The drawing under review shows one solid part. Ordinate dimensions are in mm from its lowest x, y, z. Give positions to 0.01 mm unless a question says otherwise; leave off trailing zeros. Loops run counter-clockwise (first coordinate to the right, second up) from the corner with the lowest first, then second, coordinate; pieces in that order, holes last. Notation, with made-up numbers: M 35,-31.75 L 91,-31.75 A17 cw 91,-14.75 Z; hole C 14.25,26 d1. An arc over 180 degrees is marked long. Put each result on its own line as item: value. Start each with the question number.
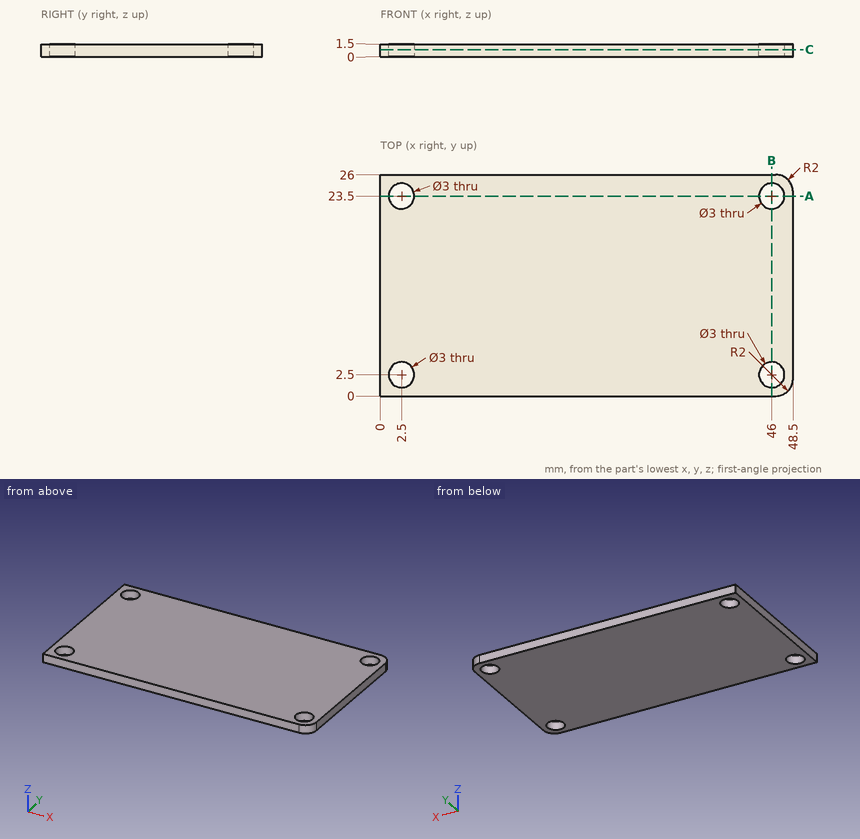
(1) We need section A-A, the plane y = 23.5. Write out the cut boundary in (x, z), plus the area to 4 significant figures.
(2) To check wall thickness, follow L1, parallel to Y at x = 46, z = 1.1; L2, parallel to X at y = 24.5, z = 0.4; L3, parallel to Y at x = 45.5, z = 1.3. State the ranges of each line that lie inside material, in increasing order. Write a range as [from, to].
(3) We need section C-C, the plane z = 0.85. Write out the cut boundary in (x, y), plus the area to 3 significant figures.
(4) We need section B-B, the plane x = 46. Write out the cut boundary in (y, z).
Check sheet entries:
1. outline: M 0,0 L 1,0 L 1,1.5 L 0,1.5 Z; M 4,0 L 44.5,0 L 44.5,1.5 L 4,1.5 Z; M 47.5,0 L 48.5,0 L 48.5,1.5 L 47.5,1.5 Z
1. area: 63.75 mm²
2. L1: y = [0, 1], [4, 22], [25, 26]
2. L2: x = [0, 1.38], [3.62, 44.88], [47.12, 48.44]
2. L3: y = [0, 1.09], [3.91, 22.09], [24.91, 26]
3. outline: M 0,0 L 46.5,0 A2 ccw 48.5,2 L 48.5,24 A2 ccw 46.5,26 L 0,26 Z; hole C 2.5,2.5 d3; hole C 2.5,23.5 d3; hole C 46,2.5 d3; hole C 46,23.5 d3
3. area: 1,230 mm²
4. outline: M 0,0 L 1,0 L 1,1.5 L 0,1.5 Z; M 4,0 L 22,0 L 22,1.5 L 4,1.5 Z; M 25,0 L 26,0 L 26,1.5 L 25,1.5 Z
